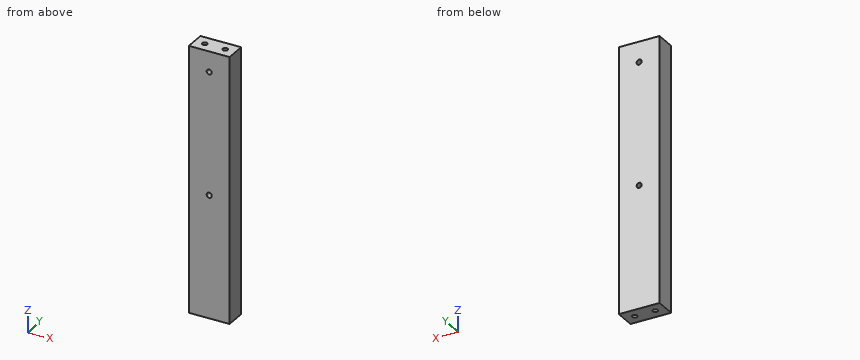
Autodesk Inventor part; units mm, degrees
ref_plane "YZ Plane" through (0, 0, 0) normal (1, 0, 0) x (0, 1, 0)
ref_plane "XZ Plane" through (0, 0, 0) normal (0, 1, 0) x (-1, 0, 0)
ref_plane "XY Plane" through (0, 0, 0) normal (0, 0, 1) x (1, 0, 0)
sketch "Sketch1" plane through (0, 0, 0) normal (0, 1, 0) x (-1, 0, 0)
  line L0 (28.8109, 92.1657) -> (-21.9891, 92.1657)
  line L1 (-21.9891, 92.1657) -> (-21.9891, -238.0343)
  line L2 (-21.9891, -238.0343) -> (28.8109, -238.0343)
  line L3 (28.8109, -238.0343) -> (28.8109, 92.1657)
  point P0 (0, 0)
  dimension "d0" = 50.8
  dimension "d1" = 330.2
extrude "Extrusion1" add sketch "Sketch1" along normal blind 25.4
sketch "Sketch2" plane through (-28.8109, 0, 92.1657) normal (0, 0, 1) x (1, 0, 0)
  line L0 (0, 0) -> (0, 25.4)
  line L1 (0, 12.7) -> (50.8, 12.7) construction
  line L2 (50.8, 0) -> (50.8, 25.4)
  circle A0 centre (12.7, 12.7) radius 3.175
  circle A1 centre (38.1, 12.7) radius 3.175
  line L3 (50.8, 25.4) -> (0, 25.4) construction
  line L4 (25.4, 25.4) -> (25.4, 0) construction
  line L5 (50.8, 0) -> (0, 0) construction
  point P0 (28.8109, 0)
  dimension "d4" = 6.35
  dimension "d5" = 6.35
  dimension "d6" = 12.7
  dimension "d7" = 12.7
extrude "Extrusion2" cut sketch "Sketch2" against normal blind 25.4
sketch "Sketch3" plane through (21.9891, 0, -238.0343) normal (0, 0, -1) x (-1, 0, 0)
  line L0 (0, 0) -> (0, 25.4) construction
  line L1 (0, 12.7) -> (50.8, 12.7) construction
  line L2 (50.8, 0) -> (50.8, 25.4) construction
  line L3 (50.8, 25.4) -> (0, 25.4) construction
  line L4 (25.4, 25.4) -> (25.4, 0) construction
  line L5 (50.8, 0) -> (0, 0) construction
  circle A0 centre (12.7, 12.7) radius 3.175
  circle A1 centre (12.7, 12.7) radius 3.175 construction
  circle A2 centre (38.1, 12.7) radius 3.175
  circle A3 centre (38.1, 12.7) radius 3.175 construction
  point P0 (21.9891, 0)
extrude "Extrusion3" cut sketch "Sketch3" against normal blind 25.4
sketch "Sketch4" plane through (0, 25.4, 0) normal (0, 1, 0) x (1, 0, 0)
  line L0 (-28.8109, -92.1657) -> (21.9891, -92.1657) construction
  line L1 (-3.4109, -92.1657) -> (-3.4109, 238.0343) construction
  line L2 (21.9891, 238.0343) -> (-28.8109, 238.0343) construction
  line L3 (-28.8109, 238.0343) -> (-28.8109, -92.1657) construction
  line L4 (-28.8109, 72.9343) -> (21.9891, 72.9343) construction
  line L5 (21.9891, -92.1657) -> (21.9891, 238.0343) construction
  circle A0 centre (-3.4109, -66.7657) radius 3.175
  circle A1 centre (-3.4109, 85.6343) radius 3.175
  point P0 (0, 0)
  dimension "d12" = 6.35
  dimension "d13" = 152.4
  dimension "d14" = 25.4
extrude "Extrusion4" cut sketch "Sketch4" against normal through all
properties part number "chair support"
Input: part model. Units: mm. Frame: model coordinates. Coordinates: 2 decimals unless noted, no trailing zeros. Loops run counter-clockwise (first coordinate to the right, second up) from the corner with the lowest first, then second, coordinate; pieces in that order, holes last. Notation, with made-up numbers: M 39.5,71 L 90.5,71 A32 ccw 90.5,108 Z; hole C -2,-35 d5. An arc over 180 degrees is marked long. Answer in a Markdown table with one row per item.
1. Section B-B, the plane y = 12.7. Output: boundary loops of the cut face in (x, z) (3 decimals), then the cut area to 3 significant figures.
Response:
| item | result |
|---|---|
| outline | M -28.811,-238.034 L -19.286,-238.034 L -19.286,-212.634 L -12.936,-212.634 L -12.936,-238.034 L 6.114,-238.034 L 6.114,-212.634 L 12.464,-212.634 L 12.464,-238.034 L 21.989,-238.034 L 21.989,92.166 L 12.464,92.166 L 12.464,66.766 L 6.114,66.766 L 6.114,92.166 L -12.936,92.166 L -12.936,66.766 L -19.286,66.766 L -19.286,92.166 L -28.811,92.166 Z; hole C -3.411,-85.634 d6.35; hole C -3.411,66.766 d6.35 |
| area | 16,100 mm2 |
2. First-contact query: pin 1 (5.5 mm diameter, centred on x = 9.29, y = 12.7, fed in from -Z); pin 2 (4 mm diameter, centred on x = -16.11, y = 12.7, fed in from +Z). Flat tips, straight axial feed; report the tip coordinate or a pass-through.
Response:
| item | result |
|---|---|
| pin 1 | stops at z = -212.63 |
| pin 2 | stops at z = 66.77 |
3. Section A-A, the plane x = -3. Output: boundary loops of the cut face in (y, z).
Response:
| item | result |
|---|---|
| outline | M 0,-238.03 L 25.4,-238.03 L 25.4,-88.78 L 0,-88.78 Z; M 0,-82.49 L 25.4,-82.49 L 25.4,63.62 L 0,63.62 Z; M 0,69.91 L 25.4,69.91 L 25.4,92.17 L 0,92.17 Z |
4. Material intervals for line 1 (Y direction, x = 6.5, z = 79); line 2 (Z direction, x = 7, y = 13.25), sorted ascending.
Response:
| item | result |
|---|---|
| line 1 | y = 0 to 11.18, 14.22 to 25.4 |
| line 2 | z = -212.63 to 66.77 |
